from build123d import *

# Parameters (mm, degrees)
SKETCH1_W             = 34.925
SKETCH1_H             = 11.1125
BOSS_EXTRUDE1_DEPTH   = 4.572
SKETCH2_W             = 1.5875
SKETCH2_H             = 11.1125
CUT_EXTRUDE1_DEPTH    = 2.286
BOSS_EXTRUDE2_DEPTH   = 2.54
BOSS_EXTRUDE3_DEPTH   = 1.778
CHAMFER1_SIZE         = 0.79375
CHAMFER1_SIZE2        = 0.458271776
CHAMFER1_PART_2_SIZE  = 0.79375
CHAMFER1_PART_2_SIZE2 = 0.458271776
CHAMFER1_PART_3_SIZE  = 0.79375
CHAMFER1_PART_3_SIZE2 = 0.458271776
CHAMFER1_PART_4_SIZE  = 0.79375
CHAMFER1_PART_4_SIZE2 = 0.458271776


with BuildPart() as part:
    # Sketch1 → Boss-Extrude1 (new body)
    with BuildSketch(Plane(origin=(0, 0, 0), x_dir=(1, 0, 0), z_dir=(0, 1, 0))):
        with Locations((17.4625, 5.55625)):
            Rectangle(SKETCH1_W, SKETCH1_H)
    extrude(amount=BOSS_EXTRUDE1_DEPTH)

    # Sketch2 → Cut-Extrude1 (cut)
    with BuildSketch(Plane.XZ):
        with Locations((17.4625, -5.55625)):
            Rectangle(SKETCH2_W, SKETCH2_H)
    extrude(amount=-CUT_EXTRUDE1_DEPTH, mode=Mode.SUBTRACT)

    # Sketch3 → Boss-Extrude2 (add)
    with BuildSketch(Plane.XZ):
        with BuildLine():
            Line((5.04825, -2.808819928), (5.04825, -8.303680072))
            ThreePointArc((5.04825, -8.303680072), (2.76225, -5.55625), (5.04825, -2.808819928))
        make_face()
        with BuildLine():
            Line((6.06425, -2.808819928), (6.06425, -8.303680072))
            ThreePointArc((6.06425, -8.303680072), (8.35025, -5.55625), (6.06425, -2.808819928))
        make_face()
        with BuildLine():
            Line((28.86075, -2.808819928), (28.86075, -8.303680072))
            ThreePointArc((28.86075, -8.303680072), (26.57475, -5.55625), (28.86075, -2.808819928))
        make_face()
        with BuildLine():
            Line((29.87675, -2.808819928), (29.87675, -8.303680072))
            ThreePointArc((29.87675, -8.303680072), (32.16275, -5.55625), (29.87675, -2.808819928))
        make_face()
    extrude(amount=BOSS_EXTRUDE2_DEPTH)

    # Sketch4 → Boss-Extrude3 (add)
    with BuildSketch(Plane.XZ.offset(2.54)):
        with BuildLine():
            Line((5.04825, -2.808819928), (5.04825, -8.303680072))
            Line((5.04825, -8.303680072), (3.964944561, -8.303680072))
            ThreePointArc((3.964944561, -8.303680072), (2.38125, -5.55625), (3.964944561, -2.808819928))
            Line((3.964944561, -2.808819928), (5.04825, -2.808819928))
        make_face()
        with BuildLine():
            Line((6.06425, -2.808819928), (6.06425, -8.303680072))
            Line((6.06425, -8.303680072), (7.147555439, -8.303680072))
            ThreePointArc((7.147555439, -8.303680072), (8.73125, -5.55625), (7.147555439, -2.808819928))
            Line((7.147555439, -2.808819928), (6.06425, -2.808819928))
        make_face()
        with BuildLine():
            Line((28.86075, -2.808819928), (27.777444561, -2.808819928))
            ThreePointArc((27.777444561, -2.808819928), (26.19375, -5.55625), (27.777444561, -8.303680072))
            Line((27.777444561, -8.303680072), (28.86075, -8.303680072))
            Line((28.86075, -8.303680072), (28.86075, -2.808819928))
        make_face()
        with BuildLine():
            Line((29.87675, -2.808819928), (30.960055439, -2.808819928))
            ThreePointArc((30.960055439, -2.808819928), (32.54375, -5.55625), (30.960055439, -8.303680072))
            Line((30.960055439, -8.303680072), (29.87675, -8.303680072))
            Line((29.87675, -8.303680072), (29.87675, -2.808819928))
        make_face()
    extrude(amount=BOSS_EXTRUDE3_DEPTH)

    # Chamfer1
    chamfer1_edges = [part.edges().sort_by_distance(p)[0] for p in [
        (32.54375, -4.318, -5.55625),
    ]]
    chamfer1_side = [part.faces().sort_by_distance(p)[0] for p in [
        (32.54375, -3.429, -5.55625),
    ]]
    chamfer(chamfer1_edges, length=CHAMFER1_SIZE, length2=CHAMFER1_SIZE2, reference=chamfer1_side[0])

    # Chamfer1 part 2
    chamfer1_part_2_edges = [part.edges().sort_by_distance(p)[0] for p in [
        (26.19375, -4.318, -5.55625),
    ]]
    chamfer1_part_2_side = [part.faces().sort_by_distance(p)[0] for p in [
        (26.19375, -3.429, -5.55625),
    ]]
    chamfer(chamfer1_part_2_edges, length=CHAMFER1_PART_2_SIZE, length2=CHAMFER1_PART_2_SIZE2, reference=chamfer1_part_2_side[0])

    # Chamfer1 part 3
    chamfer1_part_3_edges = [part.edges().sort_by_distance(p)[0] for p in [
        (2.38125, -4.318, -5.55625),
    ]]
    chamfer1_part_3_side = [part.faces().sort_by_distance(p)[0] for p in [
        (2.38125, -3.429, -5.55625),
    ]]
    chamfer(chamfer1_part_3_edges, length=CHAMFER1_PART_3_SIZE, length2=CHAMFER1_PART_3_SIZE2, reference=chamfer1_part_3_side[0])

    # Chamfer1 part 4
    chamfer1_part_4_edges = [part.edges().sort_by_distance(p)[0] for p in [
        (8.73125, -4.318, -5.55625),
    ]]
    chamfer1_part_4_side = [part.faces().sort_by_distance(p)[0] for p in [
        (8.73125, -3.429, -5.55625),
    ]]
    chamfer(chamfer1_part_4_edges, length=CHAMFER1_PART_4_SIZE, length2=CHAMFER1_PART_4_SIZE2, reference=chamfer1_part_4_side[0])


solid = part.part
Verification items for the finished model (mm, model axes). A direction names the side the tool comes from. Round coordinates to 2 decimals unless told otherwise and drop trailing zeros. Write each loop counter-clockwise with the first axis right and the second up, starting at its lowest first coordinate (ties: lowest second). Pieces come first, ordered by that corner, then holes.
(1) Section check B-B (y = 1). Enter the section's corners in (x, z) (1 decimal).
Returned:
outline: (0, -11.1) - (16.7, -11.1) - (16.7, 0) - (0, 0) - close; (18.3, -11.1) - (34.9, -11.1) - (34.9, 0) - (18.3, 0) - close
(2) Mould release check, pull along Y, two halves, no side actions. Record for faces 5 (the flat face through (34.925, 2, -5)), 6 (the flat face through (2.6, -2.54, -5.5)), 7 (the flat face through (17, 4.572, -6)): pulls with the +Y half, pulls with the -Y half, needs draft (parallel to the pull), parting line crosses it, or undercut.
Returned:
face 5: needs draft
face 6: undercut
face 7: pulls with the +Y half
(3) Section check D-D (x = 17). Enter the section's corners in (y, z).
Returned:
outline: (2.29, -11.11) - (4.57, -11.11) - (4.57, 0) - (2.29, 0) - close
(4) Section check A-A (y = -1). Enter the section's corners in (x, z), plus the area to 3 significant figures.
Returned:
outline: (5.05, -8.3) - (5.05, -2.81) arc R2.79 ccw to start; (6.06, -8.3) arc R2.79 ccw to (6.06, -2.81) - close; (28.86, -8.3) - (28.86, -2.81) arc R2.79 ccw to start; (29.88, -8.3) arc R2.79 ccw to (29.88, -2.81) - close
area: 37.8 mm2
(5) Depth check by flat-ended pin: pin 1 Ø5 at (x, z) = (29.5, -10) entering from -Y; pin 2 Ø1.5 at (x, z) = (15, -7) entering from -Y; pin 3 Ø1.3 at (y, z) = (-2.5, -4.5) entering from -X; pin 4 Ø0.9 at (x, y) = (4.5, -3) entering from +Z. Enter the tip coordinate at first touch or a pass-through.
Returned:
pin 1: stops at y = -4.32
pin 2: stops at y = 0
pin 3: stops at x = 2.41
pin 4: stops at z = -2.81
(6) Material ranges on line 1 (X direction, y = 0.25, z = -3.5) (3 decimals); line 2 (Y direction, x = 2, z = -7); line 3 (Z direction, x = 31, y = -1.25), recorded low to high.
Returned:
line 1: x = 0 to 16.669, 18.256 to 34.925
line 2: y = 0 to 4.57
line 3: z = -7.82 to -3.29
(7) Access from +Z, -Z, +X, -X, +Y, -Y to the whole of each face (thin tool, end or side, straight path). Record for faces 1 (the flat face through (29.877, -2, -6)), 2 (the flat face through (4.5, -3.2, -8.304)), 3 (the cylindrical face through (26.194, -3.025, -5.51)), 4 (the cylindrical face through (26.575, -1.252, -5.611)).
Returned:
face 1: +Z, -Z, -Y
face 2: -Z, +X, -X, -Y
face 3: -Y
face 4: none
(8) Section check C-C (z = -1.5). Enter the section's corners in (x, y) (3 decimals), plus the area to 3 significant figures.
Returned:
outline: (0, 0) - (16.669, 0) - (16.669, 2.286) - (18.256, 2.286) - (18.256, 0) - (34.925, 0) - (34.925, 4.572) - (0, 4.572) - close
area: 156 mm2
